The model under review builds one solid part; all positions refer to its coordinate system, in mm. Coordinates: 2 decimals unless noted, no trailing zeros. Loops run counter-clockwise (first coordinate to the right, second up) from the corner with the lowest first, then second, coordinate; pieces in that order, holes last. Notation, with made-up numbers: (25, 72) - (46, 72) arc R21 cw to (46, 92) - close; hole circle Ø5 at (32, -0.75). An arc over 180 degrees is marked (long way). Answer in a Markdown table with one row per item. Add a question column.
(1) We need section B-B on y = 0. Write out the cut boundary in (x, z), plus the area to 3 significant figures.
(2) We need section D-D on z = 34.5. Write out the cut boundary in (x, y), plus the area to 3 significant figures.
(3) For P1, Ø3, axis at x = 14, y = 39.5, coming from the +Z side; P2, Ø20, axis at x = 0, y = 0, coming from the +Z side; P3, Ø5, axis at x = -14.5, y = 38, coming from the +Z side, all flat-tipped, find the tip position at first contact; note any pin that passes through.
(4) We need section A-A on x = 44. Write out the cut boundary in (y, z), plus the area to 3 significant figures.
(5) We need section C-C on z = 92. Write out the cut boundary in (x, y).
(6) For line 1 along X through (y, z) = (-38, 28.5); line 2 along Z through (x, y) = (-29, 44.5); line 3 along Z through (x, y) = (3, 40), list the stretches that pass through material, from the lowest coordinate up.
from build123d import *

# Parameters (mm, degrees)
SKETCH001_W  = 100
SKETCH001_H  = 100
PAD_DEPTH    = 100
SKETCH_R     = 12.5
POCKET_DEPTH = 20
FILLET_R     = 15
FILLET001_R  = 15
FILLET002_R  = 15
FILLET003_R  = 10
FILLET004_R  = 5


with BuildPart() as part:
    # Sketch001 → Pad (new body)
    with BuildSketch(Plane.XY):
        Rectangle(SKETCH001_W, SKETCH001_H)
    extrude(amount=PAD_DEPTH)

    # Sketch (on Face6 of Pad) → Pocket (cut)
    with BuildSketch(Plane.XY.offset(100)):
        Circle(SKETCH_R)
    extrude(amount=-POCKET_DEPTH, mode=Mode.SUBTRACT)

    # Fillet
    fillet_edges = [part.edges().sort_by_distance(p)[0] for p in [
        (50, -50, 50),
        (-50, -50, 50),
        (50, 50, 50),
        (-50, 50, 50),
    ]]
    fillet(fillet_edges, radius=FILLET_R)

    # Fillet001
    fillet001_edges = [part.edges().sort_by_distance(p)[0] for p in [
        (-50, 0, 100),
        (-45.606602, 45.606602, 100),
        (0, 50, 100),
        (45.606602, 45.606602, 100),
        (50, 0, 100),
        (45.606602, -45.606602, 100),
        (0, -50, 100),
        (-45.606602, -45.606602, 100),
    ]]
    fillet(fillet001_edges, radius=FILLET001_R)

    # Fillet002
    fillet002_edges = [part.edges().sort_by_distance(p)[0] for p in [
        (0, -50, 0),
        (-45.606602, -45.606602, 0),
        (-50, 0, 0),
        (-45.606602, 45.606602, 0),
        (0, 50, 0),
        (45.606602, 45.606602, 0),
        (50, 0, 0),
        (45.606602, -45.606602, 0),
    ]]
    fillet(fillet002_edges, radius=FILLET002_R)

    # Fillet003
    fillet003_edges = [part.edges().sort_by_distance(p)[0] for p in [
        (-12.5, 0, 100),
    ]]
    fillet(fillet003_edges, radius=FILLET003_R)

    # Fillet004
    fillet004_edges = [part.edges().sort_by_distance(p)[0] for p in [
        (-12.5, 0, 80),
    ]]
    fillet(fillet004_edges, radius=FILLET004_R)


solid = part.part
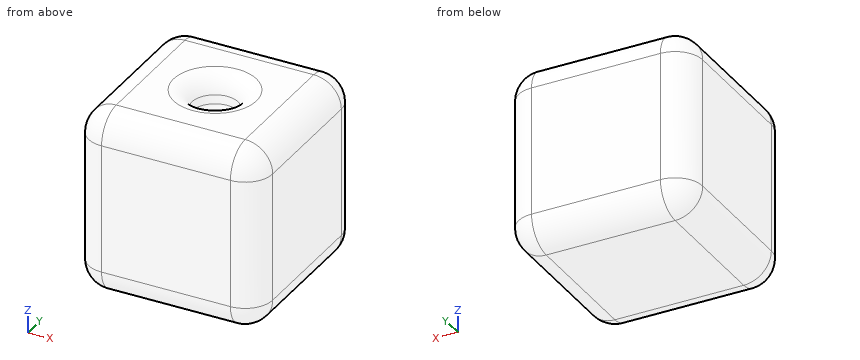
Outcome:
| question | item | result |
|---|---|---|
| 1 | outline | (-50, 15) arc R15 ccw to (-35, 0) - (35, 0) arc R15 ccw to (50, 15) - (50, 85) arc R15 ccw to (35, 100) - (22.5, 100) arc R10 ccw to (12.5, 90) - (12.5, 85) arc R5 cw to (7.5, 80) - (-7.5, 80) arc R5 cw to (-12.5, 85) - (-12.5, 90) arc R10 ccw to (-22.5, 100) - (-35, 100) arc R15 ccw to (-50, 85) - close |
| 1 | area | 9,270 mm² |
| 2 | outline | (-50, -35) arc R15 ccw to (-35, -50) - (35, -50) arc R15 ccw to (50, -35) - (50, 35) arc R15 ccw to (35, 50) - (-35, 50) arc R15 ccw to (-50, 35) - close |
| 2 | area | 9,810 mm² |
| 3 | P1 | z = 99.7 |
| 3 | P2 | z = 80.67 |
| 3 | P3 | z = 99.99 |
| 4 | outline | (-47, 15) arc R12 ccw to (-35, 3) - (35, 3) arc R12 ccw to (47, 15) - (47, 85) arc R12 ccw to (35, 97) - (-35, 97) arc R12 ccw to (-47, 85) - close |
| 4 | area | 8,710 mm² |
| 5 | outline | (-48.27, -35) arc R13.27 ccw to (-35, -48.27) - (35, -48.27) arc R13.27 ccw to (48.27, -35) - (48.27, 35) arc R13.27 ccw to (35, 48.27) - (-35, 48.27) arc R13.27 ccw to (-48.27, 35) - close; hole circle Ø25.4 at (0, 0) |
| 6 | line 1 | -49.7 to 49.7 |
| 6 | line 2 | 3.39 to 96.61 |
| 6 | line 3 | 0.86 to 99.14 |
